Read the model definition and answer for the solid it produces. Units are mm, in the model's axes. Round coordinates to 2 decimals unless told otherwise and drop trailing zeros. Loops run counter-clockwise (first coordinate to the right, second up) from the corner with the lowest first, then second, coordinate; pieces in that order, holes last. Notation, with made-up numbers: (83.5, -39.75) -> (105.5, -39.75) arc R28 cw to (105.5, -12.75) -> close; hole circle Ø5 at (-37, 53.5). An arc over 180 degrees is marked (long way). Put each result on its own line as item: value.
from build123d import *

# Parameters (mm, degrees)
SKETCH1_W                      = 330
SKETCH1_H                      = 30.4
BOSS_EXTRUDE1_DEPTH            = 3.2
M8_CLEARANCE_HOLE1_AT_2_COUNT  = 2
M8_CLEARANCE_HOLE1_AT_2_PITCH  = 201.6
M8_CLEARANCE_HOLE1_AT_3_COUNT  = 2
M8_CLEARANCE_HOLE1_AT_3_PITCH  = 100.8
F_8_0MM_DOWEL_HOLE1_AT_2_COUNT = 2
F_8_0MM_DOWEL_HOLE1_AT_2_PITCH = 167.6
M6_CLEARANCE_HOLE1_D           = 6.6


with BuildPart() as part:
    # Sketch1 → Boss-Extrude1 (new body)
    with BuildSketch(Plane(origin=(0, 0, 0), x_dir=(1, 0, 0), z_dir=(0, 1, 0))):
        Rectangle(SKETCH1_W, SKETCH1_H)
    extrude(amount=-BOSS_EXTRUDE1_DEPTH)

    # Sketch3 → M8 Clearance Hole1 (revolve, cut)
    with BuildSketch(Plane(origin=(-155, 0, -5.2), x_dir=(0, 0, 1), z_dir=(1, 0, 0))):
        Polygon((0, 0), (0, 3.2), (4.525, 3.2), (4.5, 3.175), (4.5, 0.025), (4.525, 0), align=None)
    m8_clearance_hole1 = revolve(axis=Axis((-155, 6.35, -5.2), (0, -1, 0)), mode=Mode.SUBTRACT)

    # M8 Clearance Hole1 at 2: M8 Clearance Hole1 ×2
    with Locations(*[(i * M8_CLEARANCE_HOLE1_AT_2_PITCH, 0, 0) for i in range(1, M8_CLEARANCE_HOLE1_AT_2_COUNT)]):
        add(m8_clearance_hole1, mode=Mode.SUBTRACT)

    # M8 Clearance Hole1 at 3: M8 Clearance Hole1 ×2
    with Locations(*[(i * M8_CLEARANCE_HOLE1_AT_3_PITCH, 0, 0) for i in range(1, M8_CLEARANCE_HOLE1_AT_3_COUNT)]):
        add(m8_clearance_hole1, mode=Mode.SUBTRACT)

    # Sketch5 → Ø8.0mm Dowel Hole1 (revolve, cut)
    with BuildSketch(Plane(origin=(-138, 0, -5.2), x_dir=(0, 0, 1), z_dir=(1, 0, 0))):
        Polygon((0, 0), (0, 3.2), (4.025, 3.2), (4, 3.175), (4, 0.025), (4.025, 0), align=None)
    f_8_0mm_dowel_hole1 = revolve(axis=Axis((-138, 6.35, -5.2), (0, -1, 0)), mode=Mode.SUBTRACT)

    # Ø8.0mm Dowel Hole1 at 2: Ø8.0mm Dowel Hole1 ×2
    with Locations(*[(i * F_8_0MM_DOWEL_HOLE1_AT_2_PITCH, 0, 0) for i in range(1, F_8_0MM_DOWEL_HOLE1_AT_2_COUNT)]):
        add(f_8_0mm_dowel_hole1, mode=Mode.SUBTRACT)

    # M6 Clearance Hole1 (through all)
    with Locations(Plane(origin=(0, 0, 0), x_dir=(1, 0, 0), z_dir=(0, 1, 0))):
        with Locations((142.7, 7.2), (157, -7.2)):
            Hole(M6_CLEARANCE_HOLE1_D / 2)


solid = part.part
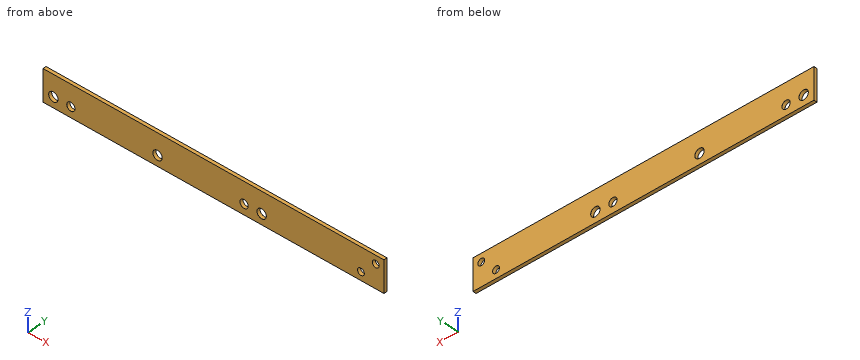
Item 1: The part is cut by section A-A (x = 29.6). Determine the outline of the cut face in (y, z) (3 decimals), then the cut area to 3 significant figures.
Derived:
outline: (-3.2, -15.2) -> (0, -15.2) -> (0, -9.225) -> (-0.025, -9.2) -> (-3.175, -9.2) -> (-3.2, -9.225) -> close; (-3.2, -1.175) -> (-3.175, -1.2) -> (-0.025, -1.2) -> (0, -1.175) -> (0, 15.2) -> (-3.2, 15.2) -> close
area: 71.7 mm^2
Item 2: The part is cut by section B-B (z = 7.2). Determine the outline of the cut face in (x, y), then the cut area to 3 significant figures.
Derived:
outline: (-165, -3.2) -> (153.7, -3.2) -> (153.7, 0) -> (-165, 0) -> close; (160.3, -3.2) -> (165, -3.2) -> (165, 0) -> (160.3, 0) -> close
area: 1,030 mm^2
Item 3: The part is cut by section D-D (x = -54.2). Determine the outline of the cut face in (y, z) (3 decimals).
Derived:
outline: (-3.2, -15.2) -> (0, -15.2) -> (0, -9.725) -> (-0.025, -9.7) -> (-3.175, -9.7) -> (-3.2, -9.725) -> close; (-3.2, -0.675) -> (-3.175, -0.7) -> (-0.025, -0.7) -> (0, -0.675) -> (0, 15.2) -> (-3.2, 15.2) -> close
Item 4: Find the intervals of material crossed by line 1 along Z through (x, y) = (-138, -1.95); line 2 along Z through (x, y) = (157, -1.6); line 3 along X through (y, z) = (-2.4, -3), in increasing order.
Derived:
line 1: z = -15.2 to -9.2, -1.2 to 15.2
line 2: z = -15.2 to 3.9, 10.5 to 15.2
line 3: x = -165 to -158.93, -151.07 to -141.34, -134.66 to -58.13, -50.27 to 26.26, 32.94 to 42.67, 50.53 to 165
Item 5: A flat-ended cylindrical pin translates along its axis: pin 1 Ø8.5 at (x, z) = (157, 7.2) entering from +Y. Find the tip coordinate at first contact, or state that the pin passes through.
Derived:
pin 1: stops at y = 0
Item 6: The part is cut by section C-C (y = -0.6). Determine the outline of the cut face in (x, z).
Derived:
outline: (-165, -15.2) -> (165, -15.2) -> (165, 15.2) -> (-165, 15.2) -> close; hole circle Ø9 at (-155, -5.2); hole circle Ø8 at (-138, -5.2); hole circle Ø9 at (-54.2, -5.2); hole circle Ø8 at (29.6, -5.2); hole circle Ø9 at (46.6, -5.2); hole circle Ø6.6 at (142.7, -7.2); hole circle Ø6.6 at (157, 7.2)
